Design review of the part shown in the three views and the two pictorial views. Dimensions are in mm from the part's minimum x, y and z. A direction names the side the tool comes from. Give positions to 0.01 mm unless a question says otherwise; leave off trailing zeros. Loops run counter-clockwise (first coordinate to the right, second up) from the corner with the lowest first, then second, coordinate; pieces in that order, holes last.
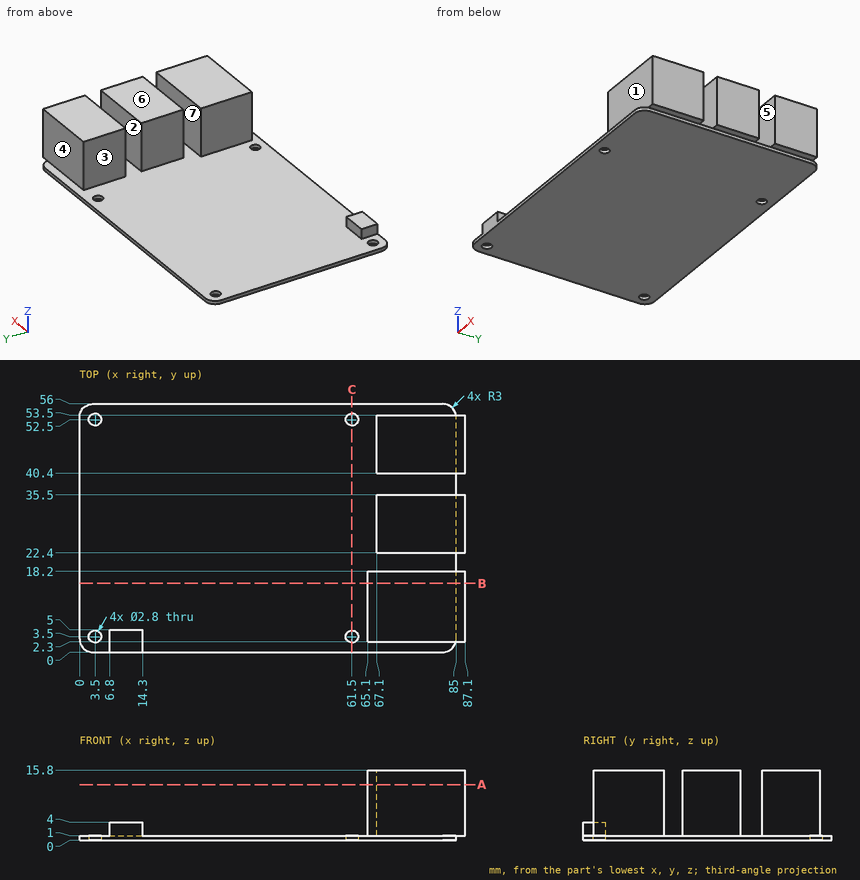
Q1. For pin 1 Ø1.5 at (y, z) = (1.5, 2) entering from +X; pin 2 Ø0.5 at (y, z) = (33, 0.5) entering from +X; pin 3 Ø6 at (x, y) = (30, 33.5) entering from -Z; pin 4 Ø1.5 at (x, z) = (74, 9.5) entering from +Y, all flat-tipped, find the tip position at first contact; note any pin that passes through.
Answers:
pin 1: stops at x = 14.3
pin 2: stops at x = 85
pin 3: stops at z = 0
pin 4: stops at y = 53.5
Q2. Consider section B-B on y = 15.5. Give the boundary of the cut face in (x, z).
Answers:
outline: (0, 0) - (85, 0) - (85, 1) - (87.1, 1) - (87.1, 15.8) - (65.1, 15.8) - (65.1, 1) - (0, 1) - close
Q3. For probe 1 along Y at (x, z) = (3.5, 0.3); probe 2 along Y at (x, z) = (69, 12.5); probe 3 along Z at (x, y) = (53.5, 51), list the stretches that pass through material, from the lowest coordinate up.
Answers:
probe 1: y = 0 to 2.1, 4.9 to 51.1, 53.9 to 56
probe 2: y = 2.3 to 18.2, 22.4 to 35.5, 40.4 to 53.5
probe 3: z = 0 to 1
Q4. Mouldability with a two-part tool opening along Y and no side actions: class the marked faces 4, 5, 6 and 7 as +Y half, -Y half, draft (parallel to the pull), parting line (faces both ways), or undercut.
Answers:
face 4: +Y half
face 5: undercut
face 6: draft
face 7: undercut
Q5. Consider section A-A on z = 12.5. Give the boundary of the cut face in (x, y), plus the area to 3 significant figures.
Answers:
outline: (65.1, 2.3) - (87.1, 2.3) - (87.1, 18.2) - (65.1, 18.2) - close; (67.1, 22.4) - (87.1, 22.4) - (87.1, 35.5) - (67.1, 35.5) - close; (67.1, 40.4) - (87.1, 40.4) - (87.1, 53.5) - (67.1, 53.5) - close
area: 874 mm2
Q6. Consider section C-C on x = 61.5. Give the boundary of the cut face in (y, z).
Answers:
outline: (0, 0) - (2.1, 0) - (2.1, 1) - (0, 1) - close; (4.9, 0) - (51.1, 0) - (51.1, 1) - (4.9, 1) - close; (53.9, 0) - (56, 0) - (56, 1) - (53.9, 1) - close
Q7. Machinability: for the marked faces 1, 2 and 3, which of the approach directions +Z, -Z, +X, -X, +Y, -Y give a long, thin tool a straight path to every point of the face, cutting with its end or side? Answer none if there is none.
Answers:
face 1: +Z, +X, -Y
face 2: +Z, +X, -X
face 3: +Z, -X, +Y
